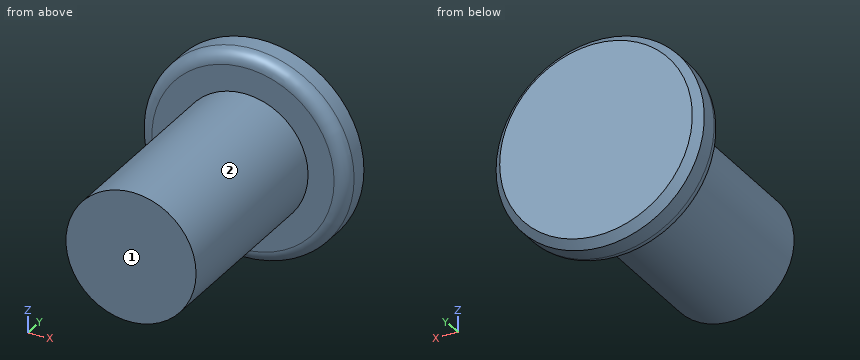
from build123d import *

# Parameters (mm, degrees)
CHAMFER_1_SIZE = 0.3
FILLET_1_R     = 0.5


with BuildPart() as part:
    # 草图2 → 旋转1 (revolve)
    with BuildSketch(Plane.XY):
        Polygon((0, -23.262759575), (4, -23.262759575), (4, -24.762759575), (2.5, -24.762759575), (2.5, -32.762759575), (0, -32.762759575), align=None)
    revolve(axis=Axis((0, -1000, 0), (0, 1, 0)))

    # 倒角1
    chamfer_1_edges = [part.edges().sort_by_distance(p)[0] for p in [
        (-4, -23.262759575, 0),
    ]]
    chamfer(chamfer_1_edges, length=CHAMFER_1_SIZE)

    # 圆角1
    fillet_1_edges = [part.edges().sort_by_distance(p)[0] for p in [
        (-4, -24.762759575, 0),
    ]]
    fillet(fillet_1_edges, radius=FILLET_1_R)


solid = part.part
Work out the finished part from the listing and answer in its coordinate system (mm). Face numbers are marked on the shaded views. A direction names the side the tool comes from. Coordinates: 2 decimals unless noted, no trailing zeros. Loops run counter-clockwise (first coordinate to the right, second up) from the corner with the lowest first, then second, coordinate; pieces in that order, holes last. Notation, with made-up numbers: M 36.5,5.5 L 61.5,5.5 A5 cw 61.5,9.5 Z; hole C 47,4 d7. An arc over 180 degrees is marked long. Answer in a Markdown table with one row per item. Add a question column.
1. Find section A-A, the plane z = 0. Write down the section's boundary in (x, y).
2. Find section C-C, the plane y = -27.25. Write down the section's boundary in (x, z).
3. Consider L1, parallel to Y at x = -3, z = 0.75; L2, parallel to X at y = -27.5, z = 0. Determine where each line is inside the solid, lowest interval first.
4. A tool of negligible diameter and unlimited length cuts with its end or side. For the marked faces 1 and 2, from which of +Z, -Z, +X, -X, +Y, -Y can it reach the whole face along a straight path? Write none if from no direction.
5. Find section B-B, the plane x = 0. Write down the section's boundary in (y, z).
6. Flat-ended cylindrical pins translate along their axes: P1, Ø2, axis at y = -27, z = 1.5, coming from the +X side; P2, Ø2, axis at x = -1, y = -30.5, coming from the -Z side; P3, Ø1.5, axis at y = -28.5, z = 3, coming from the +X side. Find the tip coordinate at first contact, or state that the pin passes through.
Reported:
| question | item | result |
|---|---|---|
| 1 | outline | M -4,-24.26 A0.5 ccw -3.5,-24.76 L -2.5,-24.76 L -2.5,-32.76 L 2.5,-32.76 L 2.5,-24.76 L 3.5,-24.76 A0.5 ccw 4,-24.26 L 4,-23.56 L 3.7,-23.26 L -3.7,-23.26 L -4,-23.56 Z |
| 2 | outline | C 0,0 d5 |
| 3 | L1 | y = -24.76 to -23.26 |
| 3 | L2 | x = -2.5 to 2.5 |
| 4 | face 1 | +Z, -Z, +X, -X, -Y |
| 4 | face 2 | -Y |
| 5 | outline | M -32.76,-2.5 L -24.76,-2.5 L -24.76,-3.5 A0.5 ccw -24.26,-4 L -23.56,-4 L -23.26,-3.7 L -23.26,3.7 L -23.56,4 L -24.26,4 A0.5 ccw -24.76,3.5 L -24.76,2.5 L -32.76,2.5 Z |
| 6 | P1 | stops at x = 2.45 |
| 6 | P2 | stops at z = -2.5 |
| 6 | P3 | stops at x = 1.09 |
